The model under review builds one solid part; all positions refer to its coordinate system, in mm. A direction names the side the tool comes from. Round coordinates to 2 decimals unless told otherwise and drop trailing zeros. Loops run counter-clockwise (first coordinate to the right, second up) from the corner with the lowest first, then second, coordinate; pieces in that order, holes last. Notation, with made-up numbers: M 27.5,33.25 L 48.5,33.25 A9 ccw 48.5,49.25 Z; hole C 70,-4 d1. An arc over 180 degrees is marked long. Return JSON: item names as keys, results as strings. Group by question number.
Q1. For faces 1 (the face through (7.605, 2.003, 0.631)), 2 (the face through (45, 0, -5)), 3 (the face through (50, -6, 0)), 4 (the face through (49, 6, 0)), 5 (the face through (45, 0, 5)), list the 3-axis set-ups (+Z, -Z, +X, -X, +Y, -Y) from which the entire face can be reached by the end or side of a thin tool; tool diameter is ignored.
Q2. Clearance check with flat-ended pins moving along their axes: pin 1 Ø1.5 at (x, z) = (44, 2) entering from +Y; pin 2 Ø5 at (x, y) = (17, 4) entering from +Z; pin 3 Ø1.6 at (x, y) = (45, -0.5) entering from -Z. State where each tip first meets the part, or that it passes through.
Q3. Consider section B-B (x = 12). State the section outline as (y, z) points.
Q4. To check wall thickness, follow line 1 along Y through (x, z) = (55, -1.05); line 2 along Y through (x, z) = (6.5, 0). State the ranges of each line that lie inside material, in increasing order.
Q5. Consider section A-A (x = 45). State the section outline as (y, z) points, and give its area (3 significant figures).
Q6. Consider section C-C (x = 38.5). State the section outline as (y, z) points.
from build123d import *
from build123d.topology import SkipClean

# Parameters (mm, degrees)
SKETCH1_R                   = 7
BOSS_EXTRUDE1_DEPTH         = 44
BOSS_EXTRUDE2_DEPTH         = 2
SKETCH3_R                   = 3
BOSS_EXTRUDE3_DEPTH         = 4
TAP_DRILL_FOR_M5_TAP1_D     = 4.2
TAP_DRILL_FOR_M5_TAP1_DEPTH = 15
TAP_DRILL_FOR_M5_TAP1_TIP   = 1.2618073
CHAMFER1_SIZE               = 1


with BuildPart() as part:
    # Sketch1 → Boss-Extrude1 (new body)
    with BuildSketch(Plane.YZ):
        with Locations(Location((0, 0, 0), (0, 0, 270))):
            Circle(SKETCH1_R)
    extrude(amount=BOSS_EXTRUDE1_DEPTH)

    # Sketch2 → Boss-Extrude2 (add)
    with SkipClean():  # the faces are left unmerged after this step: merging them gives an invalid solid
        with BuildSketch(Plane.YZ.offset(44)):
            with BuildLine():
                Line((-4.898979486, 5), (4.898979486, 5))
                ThreePointArc((4.898979486, 5), (5.4939112, 4.337849667), (6, 3.605551275))
                Line((6, 3.605551275), (6, -3.605551275))
                ThreePointArc((6, -3.605551275), (5.4939112, -4.337849667), (4.898979486, -5))
                Line((4.898979486, -5), (-4.898979486, -5))
                ThreePointArc((-4.898979486, -5), (-5.4939112, -4.337849667), (-6, -3.605551275))
                Line((-6, -3.605551275), (-6, 3.605551275))
                ThreePointArc((-6, 3.605551275), (-5.4939112, 4.337849667), (-4.898979486, 5))
            make_face()
        extrude(amount=BOSS_EXTRUDE2_DEPTH)

    # Sketch3 → Boss-Extrude3 (add, symmetric)
    with SkipClean():  # the faces are left unmerged after this step: merging them gives an invalid solid
        with BuildSketch(Plane(origin=(0, 0, 0), x_dir=(0, 1, 0), z_dir=(0, 0, 1))):
            with BuildLine():
                Line((-6, -46), (6, -46))
                Line((6, -46), (6, -55))
                ThreePointArc((6, -55), (0, -61), (-6, -55))
                Line((-6, -55), (-6, -46))
            make_face()
            with Locations(Location((0, -55, 0), (0, 0, 270))):
                Circle(SKETCH3_R, mode=Mode.SUBTRACT)
        extrude(amount=BOSS_EXTRUDE3_DEPTH, both=True)

    # Tap Drill for M5 Tap1
    with Locations(Plane(origin=(0, 0, 0), x_dir=(0, -1, 0), z_dir=(-1, 0, 0))):
        with Locations((0, 0)):
            Hole(TAP_DRILL_FOR_M5_TAP1_D / 2, depth=TAP_DRILL_FOR_M5_TAP1_DEPTH)
            with Locations((0, 0, -(TAP_DRILL_FOR_M5_TAP1_DEPTH + TAP_DRILL_FOR_M5_TAP1_TIP / 2))):  # 118° drill point
                Cone(0, TAP_DRILL_FOR_M5_TAP1_D / 2, TAP_DRILL_FOR_M5_TAP1_TIP, mode=Mode.SUBTRACT)

    # Chamfer1
    chamfer1_edges = [part.edges().sort_by_distance(p)[0] for p in [
        (0, 0, 7),
    ]]
    chamfer(chamfer1_edges, length=CHAMFER1_SIZE)


solid = part.part
Values:
{
 "1": {"face 1": "-X", "face 2": "-Z, +X, +Y, -Y", "face 3": "+Z, -Z, +X, -Y", "face 4": "+Z, -Z, +X, +Y", "face 5": "+Z, +X, +Y, -Y"},
 "2": {"pin 1": "stops at y = 6.89", "pin 2": "stops at z = 6.84", "pin 3": "stops at z = -5"},
 "3": {"outline": "C 0,0 d14; hole C 0,0 d4.2"},
 "4": {"line 1": "y = -6 to -3, 3 to 6", "line 2": "y = -7 to -2.1, 2.1 to 7"},
 "5": {"outline": "M -6,-3.61 A7 ccw -4.9,-5 L 4.9,-5 A7 ccw 6,-3.61 L 6,3.61 A7 ccw 4.9,5 L -4.9,5 A7 ccw -6,3.61 Z", "area": "117 mm2"},
 "6": {"outline": "C 0,0 d14"}
}
